Input: dimensioned drawing with shaded views. Units: mm. Origin: part minimum x, y, z. A direction names the side the tool comes from. Round coordinates to 2 decimals unless told otherwise and drop trailing zeros. Write each loop counter-clockwise with the first axis right and the second up, starting at its lowest first coordinate (ties: lowest second). Pieces come first, ordered by that corner, then holes. Notation, with made-up numbers: M 62.5,51.25 L 103.5,51.25 A22 ccw 103.5,89.25 Z; hole C 28.25,-12 d8. An arc over 180 degrees is marked long. Answer as CSV lines item,"result". Start each with the question number.
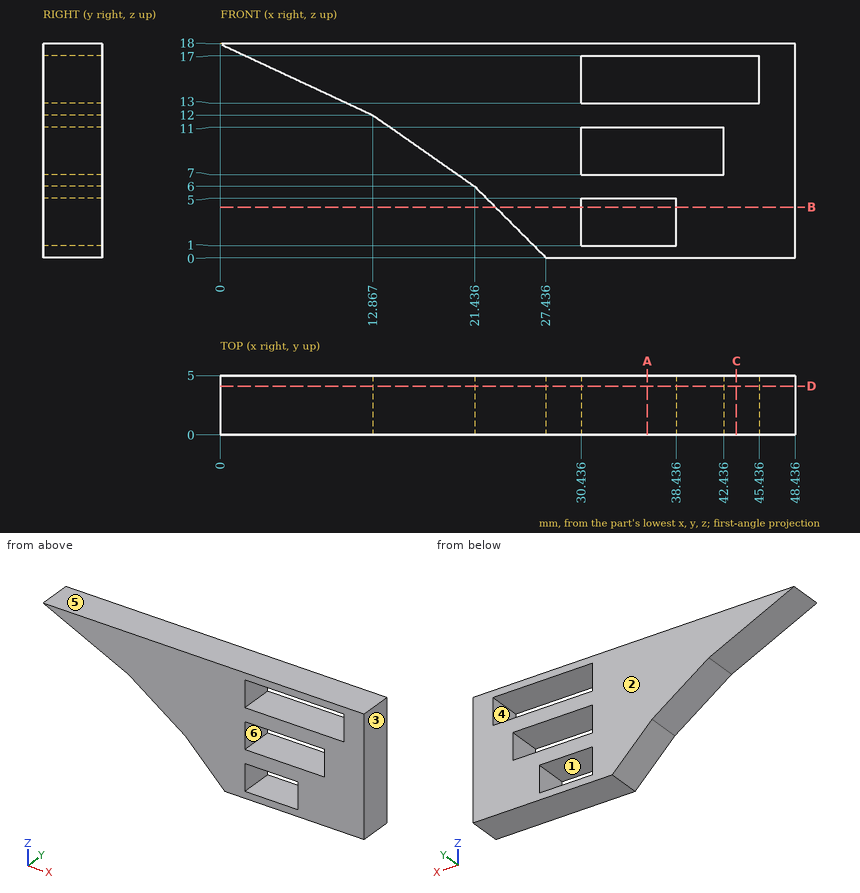
Item 1: Access query for the marked faces 1 and 2. Directions: +Z, -Z, +X, -X, +Y, -Y. A direction counts if a zero-diameter tool reaches every point of the face in a straight line with its end or side. Return the directions, or none.
Item 2: Line query: line 1 (Z direction, x = 38.5, y = 0.3); line 2 (Z direction, x = 35, y = 2.7); line 3 (Z direction, x = 45, y = 0.5). Output: solid intervals per line, ascending. Write a range as [from, to].
Item 3: Cut plane B-B, the plane z = 4.25. Return loops of the section in (x, y).
Item 4: Cut plane A-A, the plane x = 36. Return loops of the section in (y, z), plus the area to 3 significant figures.
Item 5: Draft query along Z for the marked faces 3, 4, 5 and 6. Return one class per face: +Z half, -Z half, draft (parallel to the pull), parting line (faces both ways), or undercut.
Item 6: Pin query (flat end, axial travel): pin 1 Ø1.2 at (y, z) = (1.5, 8.5) entering from -X. Return the tip coordinate at first contact, or that it passes through.
Item 7: Cut plane D-D, the plane y = 4.1. Return loops of the section in (x, z).
Item 8: Cut plane C-C, the plane x = 43.5. Return loops of the section in (y, z), plus the area to 3 significant figures.
Results list:
1,face 1,"+Y, -Y"
1,face 2,"+Z, -Z, +X, -X, +Y"
2,line 1,"[0, 7], [11, 13], [17, 18]"
2,line 2,"[0, 1], [5, 7], [11, 13], [17, 18]"
2,line 3,"[0, 13], [17, 18]"
3,outline,"M 23.19,0 L 30.44,0 L 30.44,5 L 23.19,5 Z; M 38.44,0 L 48.44,0 L 48.44,5 L 38.44,5 Z"
4,outline,"M 0,0 L 5,0 L 5,1 L 0,1 Z; M 0,5 L 5,5 L 5,7 L 0,7 Z; M 0,11 L 5,11 L 5,13 L 0,13 Z; M 0,17 L 5,17 L 5,18 L 0,18 Z"
4,area,"30.0 mm²"
5,face 3,"draft"
5,face 4,"undercut"
5,face 5,"+Z half"
5,face 6,"undercut"
6,pin 1,"x = 17.01"
7,outline,"M 0,18 L 12.87,12 L 21.44,6 L 27.44,0 L 48.44,0 L 48.44,18 Z; hole M 30.44,1 L 38.44,1 L 38.44,5 L 30.44,5 Z; hole M 30.44,7 L 42.44,7 L 42.44,11 L 30.44,11 Z; hole M 30.44,13 L 45.44,13 L 45.44,17 L 30.44,17 Z"
8,outline,"M 0,0 L 5,0 L 5,13 L 0,13 Z; M 0,17 L 5,17 L 5,18 L 0,18 Z"
8,area,"70.0 mm²"
